Could you check a few things on this model? Use its own coordinates, in mm. A direction names the side the tool comes from. Round coordinates to 2 decimals unless told otherwise and drop trailing zeros. Write each loop counter-clockwise with the first axis right and the second up, starting at its lowest first coordinate (ties: lowest second). Pieces come first, ordered by that corner, then holes. Notation, with made-up numbers: (88.5, 16) -> (99.5, 16) arc R15 cw to (99.5, 21) -> close; hole circle Ø1 at (49.5, 12). An arc over 180 degrees is marked (long way). Answer as CSV lines item,"result". Start each with the question number.
Q1. Imagine slicing it at B-B on y = 0.5. Please give me the cut outline in (x, z).
Q2. If we mould it in two halves opening along X, with no side actions, what happens to faces 5 (the flat face through (10.4, -2.5, -4.5)), 6 (the cylindrical face through (12, -2, -9)), 7 (the flat face through (12.5, -14, 8))? For each: pulls with the +X half, pulls with the -X half, needs draft (parallel to the pull), parting line crosses it, or undercut.
Q3. For faces 1 (the cylindrical face through (-10.5, -22.5, 7.5)), 2 (the flat face through (8, -2, -3)), 3 (the cylindrical face through (12, -2.5, -6.6)), 4 (the cylindrical face through (-10.5, -6, 7.5)), which set-ups out of +Z, -Z, +X, -X, +Y, -Y let a thin tool reach every point of the face, with its end or its side?
Q4. Imagine slicing it at C-C on x = -13. Please give me the cut outline in (y, z).
Q5. Will these pins go through, and if not, where does the flat tip stop? pin 1 Ø6.5 at (x, z) = (12.5, -3) entering from +Y; pin 2 Ø6 at (x, y) = (-12.5, -9.5) entering from -Z; pin 3 Ø0.5 at (y, z) = (-1.5, -4.5) entering from -X; pin 4 Ø5.5 at (y, z) = (-14.5, 8) entering from +X.
Q6. Imagine slicing it at A-A on z = 6.5. Please give me the cut outline in (x, y), and give its area (3 significant figures).
Q7. If I drill on line 1 (Y direction, x = -10.5, z = 6.25); line 2 (Y direction, x = -10.5, z = 3.5); line 3 (X direction, y = -21, z = 7.25), over which ranges is the centre line in solid material (lowest first)? Write a range as [from, to].
Q8. Imagine slicing it at D-D on y = -11.5. Please give me the cut outline in (x, z), and give its area (3 significant figures).
from build123d import *

# Parameters (mm, degrees)
SKETCH1_W           = 60
SKETCH1_H           = 5
BOSS_EXTRUDE1_DEPTH = 5
SKETCH1_3_W         = 60
SKETCH1_3_H         = 5
BOSS_EXTRUDE2_DEPTH = 5
SKETCH1_4_W         = 60
SKETCH1_4_H         = 5
BOSS_EXTRUDE3_DEPTH = 30
SKETCH2_W           = 10
SKETCH2_H           = 35
SKETCH2_R           = 1
CUT_EXTRUDE1_DEPTH  = 45.676615807
BOSS_EXTRUDE4_START = 5
SKETCH2_3_R         = 1
BOSS_EXTRUDE4_DEPTH = 5


with BuildPart() as part:
    # Sketch1 → Boss-Extrude1 (new body)
    # profile 1 of 2: a face of its own
    with BuildSketch(Plane(origin=(0, 0, 0), x_dir=(1, 0, 0), z_dir=(0, 1, 0))):
        with Locations((0, -2.5)):
            Rectangle(SKETCH1_W, SKETCH1_H)
    # profile 2 of 2: a face of its own
    with BuildSketch(Plane(origin=(0, 0, 0), x_dir=(1, 0, 0), z_dir=(0, 1, 0))):
        with BuildLine():
            Line((-16, 5), (-16, 0))
            Line((-16, 0), (-8, 0))
            Line((-8, 0), (-8, 5))
            ThreePointArc((-8, 5), (-12, 9), (-16, 5))
        make_face()
        with BuildLine():
            Line((-13.6, 4), (-13.6, 5))
            ThreePointArc((-13.6, 5), (-12, 6.6), (-10.4, 5))
            Line((-10.4, 5), (-10.4, 4))
            ThreePointArc((-10.4, 4), (-12, 2.4), (-13.6, 4))
        make_face(mode=Mode.SUBTRACT)
    extrude(amount=BOSS_EXTRUDE1_DEPTH)

    # Sketch1_3 → Boss-Extrude2 (add)
    # profile 1 of 2: a face of its own
    with BuildSketch(Plane(origin=(0, 0, 0), x_dir=(1, 0, 0), z_dir=(0, 1, 0))):
        with BuildLine():
            Line((8, 5), (8, 0))
            Line((8, 0), (16, 0))
            Line((16, 0), (16, 5))
            ThreePointArc((16, 5), (12, 9), (8, 5))
        make_face()
        with BuildLine():
            ThreePointArc((10.4, 5), (12, 6.6), (13.6, 5))
            Line((13.6, 5), (13.6, 4))
            ThreePointArc((13.6, 4), (12, 2.4), (10.4, 4))
            Line((10.4, 4), (10.4, 5))
        make_face(mode=Mode.SUBTRACT)
    # profile 2 of 2: a face of its own
    with BuildSketch(Plane(origin=(0, 0, 0), x_dir=(1, 0, 0), z_dir=(0, 1, 0))):
        with Locations((0, -2.5)):
            Rectangle(SKETCH1_3_W, SKETCH1_3_H)
    extrude(amount=-BOSS_EXTRUDE2_DEPTH)

    # Sketch1_4 → Boss-Extrude3 (add)
    with BuildSketch(Plane(origin=(0, 0, 0), x_dir=(1, 0, 0), z_dir=(0, 1, 0))):
        with Locations((0, -2.5)):
            Rectangle(SKETCH1_4_W, SKETCH1_4_H)
    extrude(amount=-BOSS_EXTRUDE3_DEPTH)

    # Sketch2 → Cut-Extrude1 (cut, through all)
    with BuildSketch(Plane.XY.offset(5)):
        with Locations((-25, -12.5)):
            Rectangle(SKETCH2_W, SKETCH2_H)
        with Locations((25, -12.5)):
            Rectangle(SKETCH2_W, SKETCH2_H)
        with Locations((-10.5, -8)):
            Circle(SKETCH2_R)
        with Locations((-10.5, -20.5)):
            Circle(SKETCH2_R)
        with Locations((10.5, -8)):
            Circle(SKETCH2_R)
        with Locations((10.5, -20.5)):
            Circle(SKETCH2_R)
    extrude(amount=-CUT_EXTRUDE1_DEPTH, mode=Mode.SUBTRACT)

    # Sketch2_3 → Boss-Extrude4 (add)
    # profile 1 of 2: a face of its own
    with BuildSketch(Plane.XY.offset(5).offset(BOSS_EXTRUDE4_START)):
        with BuildLine():
            Line((-12.5, -8), (-12.5, -20.5))
            ThreePointArc((-12.5, -20.5), (-10.5, -22.5), (-8.5, -20.5))
            Line((-8.5, -20.5), (-8.5, -8))
            ThreePointArc((-8.5, -8), (-10.5, -6), (-12.5, -8))
        make_face()
        with Locations((-10.5, -8)):
            Circle(SKETCH2_3_R, mode=Mode.SUBTRACT)
        with Locations((-10.5, -20.5)):
            Circle(SKETCH2_3_R, mode=Mode.SUBTRACT)
    # profile 2 of 2: a face of its own
    with BuildSketch(Plane.XY.offset(5).offset(BOSS_EXTRUDE4_START)):
        with BuildLine():
            ThreePointArc((12.5, -20.5), (10.5, -22.5), (8.5, -20.5))
            Line((8.5, -20.5), (8.5, -8))
            ThreePointArc((8.5, -8), (10.5, -6), (12.5, -8))
            Line((12.5, -8), (12.5, -20.5))
        make_face()
        with Locations((10.5, -20.5)):
            Circle(SKETCH2_3_R, mode=Mode.SUBTRACT)
        with Locations((10.5, -8)):
            Circle(SKETCH2_3_R, mode=Mode.SUBTRACT)
    extrude(amount=-BOSS_EXTRUDE4_DEPTH)


solid = part.part
Checks:
1,outline,"(-20, 0) -> (-16, 0) -> (-16, -5) arc R4 ccw to (-8, -5) -> (-8, 0) -> (20, 0) -> (20, 5) -> (-20, 5) -> close; hole (-13.6, -5) arc R1.6 ccw to (-10.4, -5) -> (-10.4, -4) arc R1.6 ccw to (-13.6, -4) -> close"
2,face 5,"undercut"
2,face 6,"parting line crosses it"
2,face 7,"pulls with the +X half"
3,face 1,"+Z, -Y"
3,face 2,"-Z, -X, +Y, -Y"
3,face 3,"+Y, -Y"
3,face 4,"+Z, +Y"
4,outline,"(-30, 0) -> (0, 0) -> (0, -2.75) -> (5, -2.75) -> (5, 5) -> (-30, 5) -> close; (0, -8.87) -> (5, -8.87) -> (5, -6.25) -> (0, -6.25) -> close"
5,pin 1,"y = 5"
5,pin 2,"z = 0"
5,pin 3,"x = 8"
5,pin 4,"x = 12.5"
6,outline,"(-12.5, -20.5) arc R2 ccw to (-8.5, -20.5) -> (-8.5, -8) arc R2 ccw to (-12.5, -8) -> close; (8.5, -20.5) arc R2 ccw to (12.5, -20.5) -> (12.5, -8) arc R2 ccw to (8.5, -8) -> close; hole circle Ø2 at (-10.5, -20.5); hole circle Ø2 at (-10.5, -8); hole circle Ø2 at (10.5, -20.5); hole circle Ø2 at (10.5, -8)"
6,area,"113 mm^2"
7,line 1,"[-22.5, -21.5], [-19.5, -9], [-7, -6]"
7,line 2,"[-30, -21.5], [-19.5, -9], [-7, 5]"
7,line 3,"[-12.44, -11.37], [-9.63, -8.56], [8.56, 9.63], [11.37, 12.44]"
8,outline,"(-20, 0) -> (20, 0) -> (20, 5) -> (12.5, 5) -> (12.5, 10) -> (8.5, 10) -> (8.5, 5) -> (-8.5, 5) -> (-8.5, 10) -> (-12.5, 10) -> (-12.5, 5) -> (-20, 5) -> close"
8,area,"240 mm^2"
